Source: CAD feature listing. Evaluate the final solid. Frame: model axes, mm. A direction names the side the tool comes from. Round coordinates to 2 decimals unless told otherwise and drop trailing zeros. Loops run counter-clockwise (first coordinate to the right, second up) from the corner with the lowest first, then second, coordinate; pieces in that order, holes last.
(1) Section B-B, the plane y = 18.25. Return the cut outline in (x, z).
(2) Mould query, pull axis Z, two halves, no side actions, for faces 5 (the flat face through (-55.6, 5.7, -20.06)), 6 (the flat face through (0, 0, -4)), 7 (the flat face through (13.785, 3, -25)), 8 (the flat face through (0, 3, 76)). Classes: pulls with the +Z half, pulls with the -Z half, needs draft (parallel to the pull), parting line crosses it, or undercut.
(3) Material intervals for probe 1 along X at (y, z) = (1.8, 12.97); probe 2 along Y at (x, z) = (57.5, -16); probe 3 along X at (y, z) = (1.75, -42.5), sorted ascending.
(4) Section A-A, the plane z = -18. Return the cut outline in (x, y).
(5) Set-up query: faces 1 (the flat face through (16.06, 3, 44)), 2 (the flat face through (-13.785, 3, -25)), 3 (the flat face through (16.06, 3, -52)), 4 (the flat face through (-70, 13, -4)). Return all of +Z, -Z, +X, -X, +Y, -Y with unobstructed straight access to the full face (end or side cutting, diameter ignored); none if empty.
(6) Section C-C, the plane x = -40.5. Return the cut outline in (y, z), plus the area to 3 significant figures.
(7) First-contact query: pin 1 Ø1.8 at (y, z) = (2.5, -43) entering from -X; pin 2 Ø3 at (x, y) = (52.5, 3) entering from -Z; pin 3 Ø12 at (y, z) = (15, -7) entering from +X; pin 4 Ø8 at (y, z) = (8.5, -10) entering from +X. Flat tips, straight axial feed; report the tip coordinate or a pass-through.
```python
from build123d import *

# Parameters (mm, degrees)
SKETCH21_R           = 1.7
SKETCH21_W           = 27.57
SKETCH21_H           = 9.66
BOSS_EXTRUDE18_DEPTH = 6
SKETCH22_W           = 10
SKETCH22_H           = 32.12
BOSS_EXTRUDE19_DEPTH = 15


with BuildPart() as part:
    # Sketch21 → Boss-Extrude18 (new body)
    with BuildSketch(Plane(origin=(0, 0, 0), x_dir=(1, 0, 0), z_dir=(0, 1, 0))):
        Polygon((0, 84), (-16.06, 84), (-16.06, 20.06), (-80, 20.06), (-80, 4), (-80, -12.06), (-16.06, -12.06), (-16.06, -76), (0, -76), (16.06, -76), (16.06, -12.06), (80, -12.06), (80, 4), (80, 20.06), (16.06, 20.06), (16.06, 84), align=None)
        with Locations(Location((-12.56, 36.04, 0), (0, 0, 270))):
            Circle(SKETCH21_R, mode=Mode.SUBTRACT)
        with Locations(Location((12.56, 36.04, 0), (0, 0, 270))):
            Circle(SKETCH21_R, mode=Mode.SUBTRACT)
        with Locations(Location((12.56, -12.97, 0), (0, 0, 270))):
            Circle(SKETCH21_R, mode=Mode.SUBTRACT)
        with Locations(Location((-12.56, -12.97, 0), (0, 0, 270))):
            Circle(SKETCH21_R, mode=Mode.SUBTRACT)
        with Locations((0, 25.47)):
            Rectangle(SKETCH21_W, SKETCH21_H, mode=Mode.SUBTRACT)
    extrude(amount=BOSS_EXTRUDE18_DEPTH)

    # Sketch22 → Boss-Extrude19 (add)
    with BuildSketch(Plane(origin=(0, 6, 0), x_dir=(1, 0, 0), z_dir=(0, 1, 0))):
        with Locations((-75, 4)):
            Rectangle(SKETCH22_W, SKETCH22_H)
    extrude(amount=BOSS_EXTRUDE19_DEPTH)


solid = part.part
```
Output values:
1. outline: (-80, -20.06) - (-70, -20.06) - (-70, 12.06) - (-80, 12.06) - close
2. face 5: pulls with the -Z half
2. face 6: needs draft
2. face 7: undercut
2. face 8: pulls with the +Z half
3. probe 1: x = -16.06 to -14.26, -10.86 to 10.86, 14.26 to 16.06
3. probe 2: y = 0 to 6
3. probe 3: x = -16.06 to 16.06
4. outline: (-80, 0) - (80, 0) - (80, 6) - (-70, 6) - (-70, 21) - (-80, 21) - close
5. face 1: +Z, +X, +Y, -Y
5. face 2: +Y, -Y
5. face 3: -Z, +X, +Y, -Y
5. face 4: +Z, -Z, +X, +Y
6. outline: (0, -20.06) - (6, -20.06) - (6, 12.06) - (0, 12.06) - close
6. area: 193 mm2
7. pin 1: stops at x = -16.06
7. pin 2: stops at z = -20.06
7. pin 3: stops at x = -70
7. pin 4: stops at x = 80
